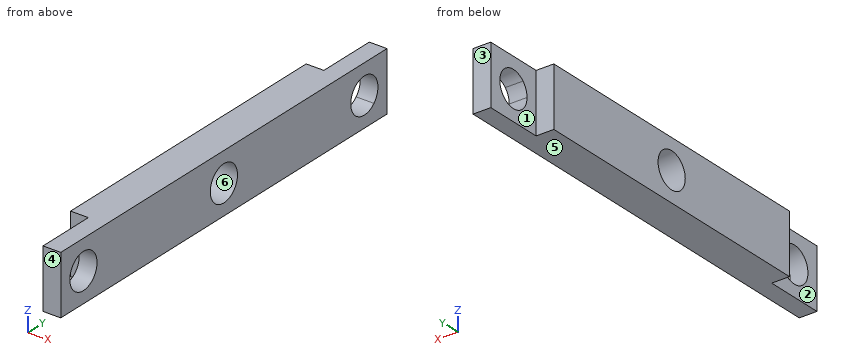
```python
from build123d import *

# Parameters (mm, degrees)
F0_W     = 228.6
F0_H     = 31.75
F1_DEPTH = 19.05
F2_W     = 31.75
F2_H     = 31.75
F3_DEPTH = 9.525
F4_R     = 9.525
F5_DEPTH = 25.4
F6_R     = 9.525
F7_DEPTH = 25.4


with BuildPart() as f1:
    # F0 (on Right) → F1 (new body)
    with BuildSketch(Plane.YZ):
        Rectangle(F0_W, F0_H)
    extrude(amount=F1_DEPTH)

    # F2 (on face) → F3 (cut)
    with BuildSketch(Plane(origin=(0, 0, 0), x_dir=(0, -1, 0), z_dir=(-1, 0, 0))):
        with Locations((-98.425, 0)):
            Rectangle(F2_W, F2_H)
        with Locations((98.425, 0)):
            Rectangle(F2_W, F2_H)
    extrude(amount=-F3_DEPTH, mode=Mode.SUBTRACT)

    # F4 (on face) → F5 (cut)
    with BuildSketch(Plane(origin=(9.525, 0, 0), x_dir=(0, -1, 0), z_dir=(-1, 0, 0))):
        with BuildLine():
            ThreePointArc((-91.689808, 6.735192), (-105.160192, 6.735192), (-105.160192, -6.735192))
            Line((-105.160192, -6.735192), (-91.689808, 6.735192))
        make_face()
        with BuildLine():
            Line((-91.689808, 6.735192), (-105.160192, -6.735192))
            ThreePointArc((-105.160192, -6.735192), (-94.77994, -8.799953), (-88.9, 0))
            ThreePointArc((-88.9, 0), (-89.625047, 3.64506), (-91.689808, 6.735192))
        make_face()
        with Locations((98.425, 0)):
            Circle(F4_R)
    extrude(amount=-F5_DEPTH, mode=Mode.SUBTRACT)

    # F6 (on face) → F7 (cut)
    with BuildSketch(Plane(origin=(0, 0, 0), x_dir=(0, -1, 0), z_dir=(-1, 0, 0))):
        Circle(F6_R)
    extrude(amount=-F7_DEPTH, mode=Mode.SUBTRACT)


solid = f1.part
```
Could you check a few things on this model? Use its own coordinates, in mm. Face numbers are marked on the shaded views. A direction names the side the tool comes from. Coordinates: 2 decimals unless noted, no trailing zeros. Order: outer loops, then holes, each group sorted by start corner. A loop starts at its lowest first (then second) coordinate and runs counter-clockwise, first axis right, second up. Notation, with made-up numbers: M -14.75,82.5 L -0.75,82.5 A12 cw -0.75,89.5 Z; hole C 24.25,6.5 d11. An arc over 180 degrees is marked long. Use one line per item in the form item = value. Start each with the question number.
1. Please list where these lines run through material, in increasing order: line 1 (Z direction, x = 14, y = 0) (3 decimals); line 2 (Y direction, x = 16.25, z = -5.5); line 3 (Y direction, x = 18, z = -3).
2. Suppose I cut it at B-B on y = 0. Write out the boundary of the cut face in (x, z) (3 decimals), then the cut area to 3 significant figures.
3. Suppose I cut it at A-A on x = 14.5. Write out the boundary of the cut face in (y, z) (3 decimals), then the cut area to 3 significant figures.
4. On a 3-axis mill with a long thin cutter (end or side, diameter ignored), from which of +Z, -Z, +X, -X, +Y, -Y can I reach the whole of each face in a straight line? I mean the marked faces 1, 2 and 3. Say none if no direction works.
5. We'd pull the mould along Y, two halves only. Please class the marked faces 4, 5 and 6: +Y half, -Y half, draft (parallel to the pull), parting line (faces both ways), or undercut.
6. Suppose I cut it at C-C on z = -2. Write out the boundary of the cut face in (x, y) (3 decimals), then the cut area to 3 significant figures.
7. For pin 1 (9.5 mm diameter, centred on y = -98.5, z = 5.5, fed in from -X) (3 decimals); pin 2 (1 mm diameter, centred on x = 3.5, z = -12, fed in from +Y); pin 3 (10 mm diameter, centred on x = 2.5, y = -91.5, fed in from +Z); pin 4 (5 mm diameter, centred on x = 6.5, z = 6, fed in from -Y), each with a flat end and sliding along its axis, tell me the tip position at first contact or that it passes through.
Geometry says:
q1.line_1 = -15.875 to -9.525, 9.525 to 15.875
q1.line_2 = -114.3 to -106.2, -90.65 to -7.78, 7.78 to 90.65, 106.2 to 114.3
q1.line_3 = -114.3 to -107.47, -89.38 to -9.04, 9.04 to 89.38, 107.47 to 114.3
q2.outline = M 0,-15.875 L 19.05,-15.875 L 19.05,-9.525 L 0,-9.525 Z; M 0,9.525 L 19.05,9.525 L 19.05,15.875 L 0,15.875 Z
q2.area = 242 mm^2
q3.outline = M -114.3,-15.875 L 114.3,-15.875 L 114.3,15.875 L -114.3,15.875 Z; hole C -98.425,0 d19.05; hole C 0,0 d19.05; hole M 88.9,0 A9.525 ccw long 91.69,6.735 A9.525 ccw Z
q3.area = 6,400 mm^2
q4.face_1 = +Z, -Z, -X, +Y
q4.face_2 = +Z, -Z, -X, -Y
q4.face_3 = +Z, -Z, +X, -X, +Y
q5.face_4 = -Y half
q5.face_5 = draft
q5.face_6 = undercut
q6.outline = M 0,-82.55 L 9.525,-82.55 L 9.525,-89.112 L 19.05,-89.112 L 19.05,-9.313 L 0,-9.313 Z; M 0,9.313 L 19.05,9.313 L 19.05,89.112 L 9.525,89.112 L 9.525,82.55 L 0,82.55 Z; M 9.525,-114.3 L 19.05,-114.3 L 19.05,-107.738 L 9.525,-107.738 Z; M 9.525,107.738 L 19.05,107.738 L 19.05,114.3 L 9.525,114.3 Z
q6.area = 3,040 mm^2
q7.pin_1 = 9.525
q7.pin_2 = 82.55
q7.pin_3 = through
q7.pin_4 = -82.55
